from build123d import *

# Parameters (mm, degrees)
SKETCH_1_R       = 11.95
EXTRUDE_1_DEPTH  = 18.7
EXTRUDE_START    = -16.2
EXTRUDE_8_DEPTH  = 16.2
EXTRUDE_START_2  = -0.8
SKETCH_3_R       = 2
EXTRUDE_9_DEPTH  = 0.8
SKETCH_4_R       = 3.85
EXTRUDE_10_DEPTH = 1.5
SKETCH_5_R       = 2.5
EXTRUDE_11_DEPTH = 8.9


with BuildPart() as part:
    # 草图1 → 凸台-拉伸1 (new body)
    with BuildSketch(Plane(origin=(0, 0, 0), x_dir=(1, 0, 0), z_dir=(0, 1, 0))):
        with Locations(Location((0, 0, 0), (0, 0, 270))):
            Circle(SKETCH_1_R)
    extrude(amount=EXTRUDE_1_DEPTH)

    # 草图2 → 凸台-拉伸8 (add)
    with BuildSketch(Plane(origin=(0, 18.7, 0), x_dir=(1, 0, 0), z_dir=(0, 1, 0)).offset(EXTRUDE_START)):
        with BuildLine():
            ThreePointArc((9.612101747, 7.1), (11.350487123, 3.737504791), (11.95, 0))
            Line((11.95, 0), (16.35, 0))
            Line((16.35, 0), (16.35, 7.1))
            Line((16.35, 7.1), (9.612101747, 7.1))
        make_face()
        with BuildLine():
            Line((16.35, 0), (11.95, 0))
            ThreePointArc((11.95, 0), (11.350487123, -3.737504791), (9.612101747, -7.1))
            Line((9.612101747, -7.1), (16.35, -7.1))
            Line((16.35, -7.1), (16.35, 0))
        make_face()
    extrude(amount=EXTRUDE_8_DEPTH)

    # 草图3 → 凸台-拉伸9 (add)
    # profile 1 of 2: a face of its own
    with BuildSketch(Plane(origin=(0, 18.7, 0), x_dir=(1, 0, 0), z_dir=(0, 1, 0)).offset(EXTRUDE_START_2)):
        with BuildLine():
            Line((-3.5, 15.5), (-3.5, 11.42595729))
            ThreePointArc((-3.5, 11.42595729), (0, 11.95), (3.5, 11.42595729))
            Line((3.5, 11.42595729), (3.5, 15.5))
            ThreePointArc((3.5, 15.5), (0, 19), (-3.5, 15.5))
        make_face()
        with Locations(Location((0, 15.5, 0), (0, 0, 270))):
            Circle(SKETCH_3_R, mode=Mode.SUBTRACT)
    # profile 2 of 2: a face of its own
    with BuildSketch(Plane(origin=(0, 18.7, 0), x_dir=(1, 0, 0), z_dir=(0, 1, 0)).offset(EXTRUDE_START_2)):
        with BuildLine():
            Line((-3.5, -15.5), (-3.5, -11.42595729))
            ThreePointArc((-3.5, -11.42595729), (0, -11.95), (3.5, -11.42595729))
            Line((3.5, -11.42595729), (3.5, -15.5))
            ThreePointArc((3.5, -15.5), (0, -19), (-3.5, -15.5))
        make_face()
        with Locations(Location((0, -15.5, 0), (0, 0, 270))):
            Circle(SKETCH_3_R, mode=Mode.SUBTRACT)
    extrude(amount=EXTRUDE_9_DEPTH)

    # 草图4 → 凸台-拉伸10 (add)
    with BuildSketch(Plane(origin=(0, 18.7, 0), x_dir=(1, 0, 0), z_dir=(0, 1, 0))):
        with Locations(Location((-6.6, 0, 0), (0, 0, 270))):
            Circle(SKETCH_4_R)
    extrude(amount=EXTRUDE_10_DEPTH)

    # 草图5 → 凸台-拉伸11 (add)
    with BuildSketch(Plane(origin=(0, 20.2, 0), x_dir=(1, 0, 0), z_dir=(0, 1, 0))):
        with Locations(Location((-6.6, 0, 0), (0, 0, 270))):
            Circle(SKETCH_5_R)
    extrude(amount=EXTRUDE_11_DEPTH)


solid = part.part
For this review, take the finished solid that the model builds, in its own axes (mm). A direction names the side the tool comes from. Coordinates: 2 decimals unless noted, no trailing zeros. Loops run counter-clockwise (first coordinate to the right, second up) from the corner with the lowest first, then second, coordinate; pieces in that order, holes last. Notation, with made-up numbers: (-9, 45.25) -> (41, 45.25) arc R33 ccw to (41, 75.25) -> close; hole circle Ø4 at (-25.5, 24). An arc over 180 degrees is marked (long way). Write each question's results on one line, items separated by ' | '.
Q1. To check wall thickness, follow line 1 along X through (y, z) = (18.1, -15.5); line 2 along Z through (x, y) = (14, 7.75); line 3 along Y through (x, z) = (8.5, 1.5). State the ranges of each line that lie inside material, in increasing order. Write a range as [from, to].
Taken from the geometry:
line 1: [-3.5, -2], [2, 3.5] | line 2: [-7.1, 7.1] | line 3: [0, 18.7]
Q2. Add section A-A, the plane x = 0. State the section outline as (y, z) points.
Taken from the geometry:
outline: (0, -11.95) -> (17.9, -11.95) -> (17.9, -13.5) -> (18.7, -13.5) -> (18.7, 13.5) -> (17.9, 13.5) -> (17.9, 11.95) -> (0, 11.95) -> close; (17.9, -19) -> (18.7, -19) -> (18.7, -17.5) -> (17.9, -17.5) -> close; (17.9, 17.5) -> (18.7, 17.5) -> (18.7, 19) -> (17.9, 19) -> close
Q3. Add section D-D, the plane x = -10. State the section outline as (y, z) points.
Taken from the geometry:
outline: (0, -6.54) -> (18.7, -6.54) -> (18.7, -1.81) -> (20.2, -1.81) -> (20.2, 1.81) -> (18.7, 1.81) -> (18.7, 6.54) -> (0, 6.54) -> close
Q4. Mouldability with a two-part tool opening along X and no side actions: class faces 1 (the flat face through (13, 10, 7.1)), 2 (the cylindrical face through (-10.36, 19.44, -0.83)), 3 (the flat face through (16.35, 10, 0)), 4 (the cylindrical face through (-1.2, 18.3, -17.1)) as +X half, -X half, draft (parallel to the pull), parting line (faces both ways), or undercut.
Taken from the geometry:
face 1: draft | face 2: parting line | face 3: +X half | face 4: undercut
Q5. Add section C-C, the plane y = 9.75. State the section outline as (x, z) points, then the cut area to 3 significant figures.
Taken from the geometry:
outline: (9.61, -7.1) -> (16.35, -7.1) -> (16.35, 7.1) -> (9.61, 7.1) arc R11.95 ccw (long way) to start | area: 522 mm²
Q6. Add section B-B, the plane z = 0. State the section outline as (x, y) points.
Taken from the geometry:
outline: (-11.95, 0) -> (11.95, 0) -> (11.95, 2.5) -> (16.35, 2.5) -> (16.35, 18.7) -> (-2.75, 18.7) -> (-2.75, 20.2) -> (-4.1, 20.2) -> (-4.1, 29.1) -> (-9.1, 29.1) -> (-9.1, 20.2) -> (-10.45, 20.2) -> (-10.45, 18.7) -> (-11.95, 18.7) -> close
Q7. Machinability: for faces 5 (the cylindrical face through (-11.666, 9.219, -2.591)), 6 (the cylindrical face through (-4.12, 24.59, -0.33)), 7 (the cylindrical face through (0.1, 18.3, 19)), 8 (the flat face through (13, 10, -7.1)), which of the approach directions +Z, -Z, +X, -X, +Y, -Y give a long, thin tool a straight path to every point of the face, cutting with its end or side? Answer none if there is none.
Taken from the geometry:
face 5: -Y | face 6: +Y | face 7: +Z, +Y, -Y | face 8: -Z, +X, +Y, -Y
Q8. For pin 1 Ø2 at (x, y) = (12.5, 13.5) entering from -Z; pin 2 Ø12 at (x, y) = (-4, 6.5) entering from +Z; pin 3 Ø2 at (x, z) = (1, -16.5) entering from -Y, all flat-tipped, find the tip position at first contact; note any pin that passes through.
Taken from the geometry:
pin 1: z = -7.1 | pin 2: z = 11.95 | pin 3: y = 17.9
